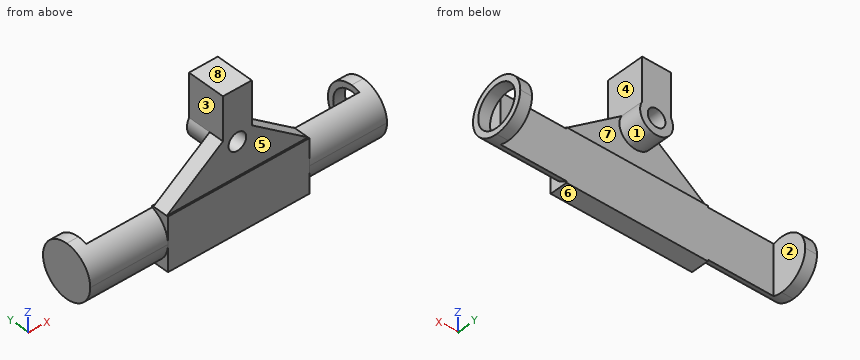
from build123d import *

# Parameters (mm, degrees)
SKETCH1_W           = 160
SKETCH1_H           = 28.575
BOSS_EXTRUDE1_DEPTH = 28.575
SKETCH3_W           = 147.3
SKETCH3_H           = 28.575
CUT_EXTRUDE3_DEPTH  = 19.05
SKETCH4_W           = 76.2
SKETCH4_H           = 8
BOSS_EXTRUDE2_DEPTH = 45.4
CUT_EXTRUDE8_DEPTH  = 124.871382326
SKETCH9_R           = 4.7625
BOSS_EXTRUDE4_DEPTH = 12.525
SKETCH10_R          = 4.7625
CUT_EXTRUDE10_DEPTH = 124.871382326
CUT_EXTRUDE11_START = -41.9
SKETCH2_OUTSIDE_W   = 111.689
SKETCH2_OUTSIDE_H   = 66.289
SKETCH2_OUTSIDE_R   = 14.2875
CUT_EXTRUDE11_DEPTH = 41.9
CUT_EXTRUDE13_START = -41.9
SKETCH13_OUTSIDE_W  = 111.689
SKETCH13_OUTSIDE_H  = 66.289
SKETCH13_OUTSIDE_R  = 14.2875
CUT_EXTRUDE13_DEPTH = 41.9
SKETCH14_R          = 11.1125
CUT_EXTRUDE14_DEPTH = 6.35


with BuildPart() as part:
    # Sketch1 → Boss-Extrude1 (new body)
    with BuildSketch(Plane(origin=(0, 0, 0), x_dir=(1, 0, 0), z_dir=(0, 1, 0))):
        with Locations((-20.782379652, -9.554800327)):
            Rectangle(SKETCH1_W, SKETCH1_H)
    extrude(amount=BOSS_EXTRUDE1_DEPTH)

    # Sketch3 → Cut-Extrude3 (cut)
    with BuildSketch(Plane(origin=(0, 28.575, 0), x_dir=(1, 0, 0), z_dir=(0, 1, 0))):
        with Locations((-20.782379652, -9.554800327)):
            Rectangle(SKETCH3_W, SKETCH3_H)
    extrude(amount=-CUT_EXTRUDE3_DEPTH, mode=Mode.SUBTRACT)

    # Sketch4 → Boss-Extrude2 (add)
    with BuildSketch(Plane.XY.offset(23.842300327)):
        with Locations((-20.782379652, 4.7625)):
            Rectangle(SKETCH4_W, SKETCH4_H)
    extrude(amount=BOSS_EXTRUDE2_DEPTH)

    # Sketch5 → Cut-Extrude8 (cut, through all)
    with BuildSketch(Plane(origin=(0, 8.7625, 0), x_dir=(1, 0, 0), z_dir=(0, 1, 0))):
        Polygon((-13.013921372, -46.075787503), (-13.013921372, -69.242300327), (17.317620348, -69.242300327), (17.317620348, -23.842300327), align=None)
        Polygon((-28.550837933, -69.242300327), (-28.550837933, -46.075787503), (-58.882379652, -23.842300327), (-58.882379652, -69.242300327), align=None)
    extrude(amount=-CUT_EXTRUDE8_DEPTH, mode=Mode.SUBTRACT)

    # Sketch9 → Boss-Extrude4 (add)
    with BuildSketch(Plane(origin=(0, 8.7625, 0), x_dir=(1, 0, 0), z_dir=(0, 1, 0))):
        with BuildLine():
            Line((-28.550837933, -46.075787503), (-28.550837933, -69.242300327))
            Line((-28.550837933, -69.242300327), (-13.013921372, -69.242300327))
            Line((-13.013921372, -69.242300327), (-13.013921372, -46.075787503))
            ThreePointArc((-13.013921372, -46.075787503), (-20.782379652, -32.954800327), (-28.550837933, -46.075787503))
        make_face()
        with Locations(Location((-20.782379652, -41.815004419, 0), (0, 0, 180))):
            Circle(SKETCH9_R, mode=Mode.SUBTRACT)
    extrude(amount=BOSS_EXTRUDE4_DEPTH)

    # Sketch10 → Cut-Extrude10 (cut, through all)
    with BuildSketch(Plane(origin=(0, 8.7625, 0), x_dir=(1, 0, 0), z_dir=(0, 1, 0))):
        with Locations(Location((-20.782379652, -41.815004419, 0), (0, 0, 180))):
            Circle(SKETCH10_R)
    extrude(amount=-CUT_EXTRUDE10_DEPTH, mode=Mode.SUBTRACT)

    # Sketch2 outside → Cut-Extrude11 (cut)
    with BuildSketch(Plane(origin=(59.217620348, 0, 0), x_dir=(0, 0, -1), z_dir=(1, 0, 0)).offset(CUT_EXTRUDE11_START)):
        with Locations((-32.2545, 14.2875)):
            Rectangle(SKETCH2_OUTSIDE_W, SKETCH2_OUTSIDE_H)
        with Locations((-9.554800327, 14.2875)):
            Circle(SKETCH2_OUTSIDE_R, mode=Mode.SUBTRACT)
    extrude(amount=CUT_EXTRUDE11_DEPTH, mode=Mode.SUBTRACT)

    # Sketch13 outside → Cut-Extrude13 (cut)
    with BuildSketch(Plane.ZY.offset(100.782379652).offset(CUT_EXTRUDE13_START)):
        with Locations((32.2545, 14.2875)):
            Rectangle(SKETCH13_OUTSIDE_W, SKETCH13_OUTSIDE_H)
        with Locations(Location((9.554800327, 14.2875, 0), (0, 0, 180))):
            Circle(SKETCH13_OUTSIDE_R, mode=Mode.SUBTRACT)
    extrude(amount=CUT_EXTRUDE13_DEPTH, mode=Mode.SUBTRACT)

    # Sketch14 → Cut-Extrude14 (cut)
    with BuildSketch(Plane(origin=(59.217620348, 0, 0), x_dir=(0, 0, -1), z_dir=(1, 0, 0))):
        with Locations((-9.554800327, 14.2875)):
            Circle(SKETCH14_R)
    extrude(amount=-CUT_EXTRUDE14_DEPTH, mode=Mode.SUBTRACT)


solid = part.part
Input: part model. Units: mm. Frame: model coordinates. Face numbers are marked on the shaded views. A direction names the side the tool comes from. Give positions to 0.01 mm unless a question says otherwise; leave off trailing zeros. Write each loop counter-clockwise with the first axis right and the second up, starting at its lowest first coordinate (ties: lowest second). Pieces come first, ordered by that corner, then holes. Notation, with made-up numbers: M 27.5,6 L 83.5,6 A16 cw 83.5,14 Z; hole C 45.5,-26.75 d5. An arc over 180 degrees is marked long. Write item = value, one per line. Start each with the question number.
1) First-contact query: pin 1 Ø10 at (x, z) = (36.5, 32.5) entering from +Y; pin 2 Ø2 at (x, z) = (-79, 4.5) entering from +Y (3 decimals); pin 3 Ø1.9 at (y, z) = (6.5, 12) entering from +X; pin 4 Ø13.5 at (x, z) = (-32, 41) entering from -Y. Flat tips, straight axial feed; report the tip coordinate or a pass-through.
2) Material intervals for line 1 along X through (y, z) = (25.5, 2); line 2 along X through (y, z) = (7.25, 58); line 3 along X through (y, z) = (12.25, 42), sorted ascending. Write a range as [from, to].
3) Draft query along Z for the marked faces 5, 6, 7 and 8. Return one class per face: +Z half, -Z half, draft (parallel to the pull), parting line (faces both ways), or undercut.
4) Cut plane A-A on y = 17. Return the cut outline in (x, z) (1 decimal), then the cut area to 3 significant figures.
5) Cut plane C-C on y = 23.75. Return the cut outline in (x, z), then the cut area to 3 significant figures.
6) Cut plane B-B on z = 44. Return the cut outline in (x, y).
7) Cut plane D-D on x = -57. Return the cut outline in (y, z) (1 decimal), then the cut area to 3 significant figures.
8) Reachability of the marked faces 1, 2, 3 and 4 from +Z, -Z, +X, -X, +Y, -Y: full face, straight path, thin tool, end or side. Return the list, or none.
Solved:
q1.pin_1 = through
q1.pin_2 = 9.525
q1.pin_3 = 52.87
q1.pin_4 = 0.76
q2.line_1 = [-100.78, -94.43], [52.87, 59.22]
q2.line_2 = [-28.55, -13.01]
q2.line_3 = [-29.64, -25.54], [-16.02, -11.92]
q3.face_5 = draft
q3.face_6 = -Z half
q3.face_7 = undercut
q3.face_8 = +Z half
q4.outline = M -100.8,-4.5 L -94.4,-4.5 L -94.4,23.6 L -100.8,23.6 Z; M -28.6,46.1 A8.9 ccw long -13,46.1 L -13,69.2 L -28.6,69.2 Z; M 52.9,-4.5 L 59.2,-4.5 L 59.2,-1.2 L 52.9,-1.2 Z; M 52.9,20.3 L 59.2,20.3 L 59.2,23.6 L 52.9,23.6 Z; hole C -20.8,41.8 d9.5
q4.area = 704 mm2
q5.outline = M -100.78,-1.15 L -94.43,-1.15 L -94.43,20.26 L -100.78,20.26 Z; M 52.87,-1.15 L 59.22,-1.15 L 59.22,3.73 L 52.87,3.73 Z; M 52.87,15.38 L 59.22,15.38 L 59.22,20.26 L 52.87,20.26 Z
q5.area = 198 mm2
q6.outline = M -31.38,0.76 L -25.01,0.76 L -25.01,21.29 L -29.37,21.29 L -29.37,8.76 L -31.38,8.76 Z; M -16.55,0.76 L -10.18,0.76 L -10.18,8.76 L -12.2,8.76 L -12.2,21.29 L -16.55,21.29 Z
q7.outline = M 0,-4.7 L 9.5,-4.7 L 9.5,23.8 L 8.8,23.8 L 8.8,25.2 L 0.8,25.2 L 0.8,23.8 L 0,23.8 Z
q7.area = 283 mm2
q8.face_1 = +Y
q8.face_2 = +Z, -Z, +Y
q8.face_3 = +Z, -X, +Y, -Y
q8.face_4 = +Z, +X, +Y, -Y
